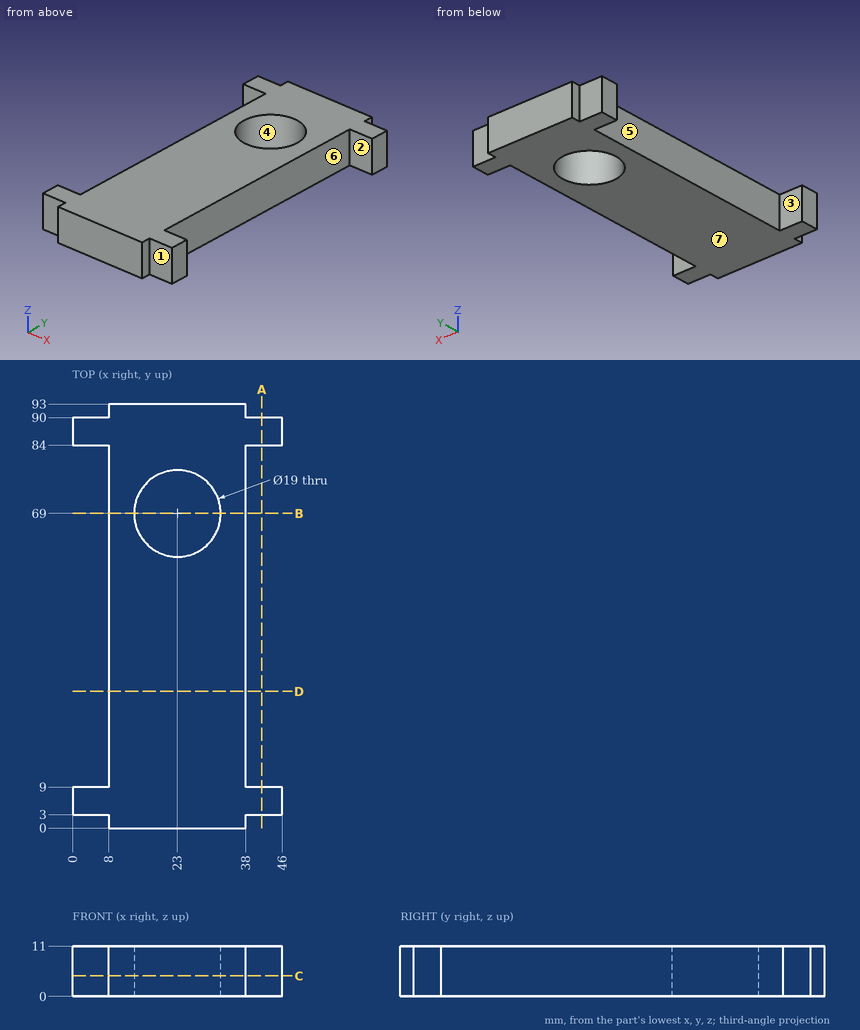
Print and shaded views of the part. All mm, measured from the part's lowest x, y and z. A direction names the side the tool comes from. Give positions to 0.01 mm unless a question says otherwise; leave off trailing zeros. Write each loop counter-clockwise with the first axis right and the second up, starting at its lowest first coordinate (ties: lowest second). Pieces come first, ordered by that corner, then holes. Notation, with made-up numbers: (-34.75, 50) - (11.25, 50) arc R26 ccw to (11.25, 87) - close; hole circle Ø2 at (66, -37.5). An arc over 180 degrees is marked (long way). One line per question, with ' | ' between items. Start each with the question number.
(1) Slice it at A-A on x = 41.5. Write the cut outline in (y, z).
(2) Two-plate mould, pull along X, no slides. Class the marked faces 4, 5, 6 and 7: +X half, -X half, draft (parallel to the pull), parting line (faces both ways), or undercut.
(3) Slice it at C-C on z = 4.5. Write the cut outline in (x, y), plus the area to 3 significant figures.
(4) Slice it at D-D on y = 30. Write the cut outline in (x, z).
(5) Wall check: line 1 along Y through (x, z) = (23, 3.5); line 2 along Y through (x, z) = (2.5, 5.75); line 3 along X through (y, z) = (58, 10). Give the ranges that are in metal, low to high. Write a range as from..to.
(6) Pin check, flat tips, straight feed: P1, Ø5.5, axis at y = 41, z = 5, coming from the -X side; P2, Ø1, axis at y = 63, z = 7.5, coming from the +X side; P3, Ø6.5, axis at x = 43.5, z = 7, coming from the -Y side. Stop position of each tip, or through.
(7) Slice it at B-B on y = 69. Write the cut outline in (x, z), plus the area to 3 significant figures.
(8) 3-axis set-ups, long thin cutter, end or side, ignore diameter. For the marked faces 1, 2 and 3: which of +Z, -Z, +X, -X, +Y, -Y reach the whole face in a straight line?
Results below:
1) outline: (3, 0) - (9, 0) - (9, 11) - (3, 11) - close; (84, 0) - (90, 0) - (90, 11) - (84, 11) - close
2) face 4: undercut | face 5: -X half | face 6: +X half | face 7: draft
3) outline: (0, 3) - (8, 3) - (8, 0) - (38, 0) - (38, 3) - (46, 3) - (46, 9) - (38, 9) - (38, 84) - (46, 84) - (46, 90) - (38, 90) - (38, 93) - (8, 93) - (8, 90) - (0, 90) - (0, 84) - (8, 84) - (8, 9) - (0, 9) - close; hole circle Ø19 at (23, 69) | area: 2,700 mm^2
4) outline: (8, 0) - (38, 0) - (38, 11) - (8, 11) - close
5) line 1: 0..59.5, 78.5..93 | line 2: 3..9, 84..90 | line 3: 8..38
6) P1: x = 8 | P2: x = 38 | P3: y = 3
7) outline: (8, 0) - (13.5, 0) - (13.5, 11) - (8, 11) - close; (32.5, 0) - (38, 0) - (38, 11) - (32.5, 11) - close | area: 121 mm^2
8) face 1: +Z, -Z, +X, -Y | face 2: +Z, -Z, +X | face 3: +Z, -Z, -X
